Could you check a few things on this model? Use its own coordinates, in mm. A direction names the side the tool comes from. Coordinates: 2 decimals unless noted, no trailing zeros. Order: outer loops, then holes, each group sorted by start corner. A loop starts at its lowest first (then second) coordinate and runs counter-clockwise, first axis right, second up.
```python
from build123d import *

# Parameters (mm, degrees)
BASPROSKE_W         = 2.8
BASPROSKE_H         = 16
TOOTHCUT_DEPTH      = 23.8
TEETHCUTS_COUNT     = 14
BORSKE_R            = 1.5
BORE_DEPTH          = 50.0000508
SKETCH_2_R          = 4.75
SKETCH_2_R_2        = 1.5
EXTRUDE_1_DEPTH     = 7
SKETCH_3_R          = 3.25
CUT_EXTRUDE_1_DEPTH = 3.5
CHAMFER_1_SIZE      = 1.5
SKETCH_4_W          = 3
SKETCH_4_H          = 9.5
CUT_EXTRUDE_2_DEPTH = 2


with BuildPart() as part:
    # BasProSke → Base-Revolve (revolve)
    with BuildSketch(Plane(origin=(0, 0, 0), x_dir=(1, 0, 0), z_dir=(0, 1, 0)), mode=Mode.PRIVATE) as base_revolve_sk:
        with Locations((1.4, 8)):
            Rectangle(BASPROSKE_W, BASPROSKE_H)
    revolve(base_revolve_sk.sketch.rotate(Axis((-10, 0, 0), (1, 0, 0)), 180), axis=Axis((-10, 0, 0), (1, 0, 0)))

    # TooCutSke → ToothCut (cut, through all)
    with BuildSketch(Plane(origin=(0, 0, 0), x_dir=(0, 0, -1), z_dir=(1, 0, 0))):
        with BuildLine():
            ThreePointArc((1.067858192, 11.449309144), (0, 11.499), (-1.067858192, 11.449309144))
            ThreePointArc((-1.067858192, 11.449309144), (-1.641684211, 13.812780716), (-3.163375005, 15.710076503))
            ThreePointArc((-3.163375005, 15.710076503), (0, 16.0254), (3.163375005, 15.710076503))
            ThreePointArc((3.163375005, 15.710076503), (1.641684211, 13.812780716), (1.067858192, 11.449309144))
        make_face()
    toothcut = extrude(amount=TOOTHCUT_DEPTH, mode=Mode.SUBTRACT)

    # TeethCuts: ToothCut ×14 about axis
    teethcuts_axis = Axis((0, 0, 0), (1, 0, 0))
    for i in range(1, TEETHCUTS_COUNT):
        add(toothcut.rotate(teethcuts_axis, i * 360 / TEETHCUTS_COUNT), mode=Mode.SUBTRACT)

    # BorSke → Bore (cut, symmetric)
    with BuildSketch(Plane(origin=(0, 0, 0), x_dir=(0, 0, -1), z_dir=(1, 0, 0))):
        with Locations(Location((0, 0, 0), (0, 0, 180))):
            Circle(BORSKE_R)
    extrude(amount=BORE_DEPTH, both=True, mode=Mode.SUBTRACT)

    # ｽｹｯﾁ2 → ﾎﾞｽ - 押し出し1 (add)
    with BuildSketch(Plane.ZY):
        with Locations(Location((0, 0, 0), (0, 0, 180))):
            Circle(SKETCH_2_R)
        Circle(SKETCH_2_R_2, mode=Mode.SUBTRACT)
    extrude(amount=EXTRUDE_1_DEPTH)

    # ｽｹｯﾁ3 → ｶｯﾄ - 押し出し1 (cut)
    with BuildSketch(Plane(origin=(2.8, 0, 0), x_dir=(0, 0, -1), z_dir=(1, 0, 0))):
        Circle(SKETCH_3_R)
    extrude(amount=-CUT_EXTRUDE_1_DEPTH, mode=Mode.SUBTRACT)

    # 面取り1
    chamfer_1_edges = [part.edges().sort_by_distance(p)[0] for p in [
        (0, 0, 4.75),
    ]]
    chamfer(chamfer_1_edges, length=CHAMFER_1_SIZE)

    # ｽｹｯﾁ4 → ｶｯﾄ - 押し出し2 (cut)
    with BuildSketch(Plane.ZY.offset(7)):
        Rectangle(SKETCH_4_W, SKETCH_4_H)
    extrude(amount=-CUT_EXTRUDE_2_DEPTH, mode=Mode.SUBTRACT)


solid = part.part
```
Item 1: Suppose I cut it at C-C (x = -3.75). List the corners of the cut face in (y, z) for me, and give its area (3 significant figures).
Item 2: I need wall thicknesses on line 1 (Y direction, x = -3.2, z = 0); line 2 (X direction, y = -3, z = 9.5); line 3 (Y direction, x = -6, z = 2). Which ranges of each line are inside material? Lowest first, please.
Item 3: Suppose I cut it at B-B (x = -6.25). List the corners of the cut face in (y, z) for me, and give its area (3 significant figures).
Item 4: Suppose I cut it at A-A (z = 0). List the corners of the cut face in (x, y) for me.
Item 5: Thinking about a two-plate mould opening in Y: for faces 1 (the face through (1.38, 1.485, 13.782)), 2 (the face through (-6, 0, -1.5)), 3 (the face through (1.42, -15.597, 3.566)), which applies, +Y half, -Y half, draft (parallel to the pull), parting line (faces both ways), or undercut?
Item 6: Which directions (+Z, -Z, +X, -X, +Y, -Y) give clear straight access to the entire face, cutting with the end or side of a thin tool? Please do faces 4 (the face through (1.38, -4.64, 13.06)), 5 (the face through (1.38, 13.77, 1.62)), 6 (the face through (1.38, -7.318, -11.773)).
Item 7: For pin 1 Ø6 at (y, z) = (0, 0) entering from -X; pin 2 Ø2.5 at (y, z) = (-1.5, 0) entering from -X; pin 3 Ø5 at (y, z) = (0, 0) entering from +X; pin 4 Ø1.6 at (x, y) = (-6, -1.5) entering from +Z, each with a flat end and sliding along its axis, tell me the tip position at first contact or that it passes through.
Geometry results:
1. outline: circle Ø9.5 at (0, 0); hole circle Ø3 at (0, 0)
1. area: 63.8 mm2
2. line 1: y = -4.75 to -1.5, 1.5 to 4.75
2. line 2: x = 0 to 2.8
2. line 3: y = -4.31 to 4.31
3. outline: (-4.51, -1.5) arc R4.75 ccw to (4.51, -1.5) - close; (-4.51, 1.5) - (4.51, 1.5) arc R4.75 ccw to start
3. area: 42.9 mm2
4. outline: (-5, -4.75) - (-1.5, -4.75) - (0, -6.25) - (0, -11.5) - (2.8, -11.5) - (2.8, -3.25) - (-0.7, -3.25) - (-0.7, -1.5) - (-5, -1.5) - close; (-5, 1.5) - (-0.7, 1.5) - (-0.7, 3.25) - (2.8, 3.25) - (2.8, 11.5) - (0, 11.5) - (0, 6.25) - (-1.5, 4.75) - (-5, 4.75) - close
5. face 1: undercut
5. face 2: draft
5. face 3: -Y half
6. face 4: +Z, +X, -X
6. face 5: +X, -X, +Y
6. face 6: +X, -X
7. pin 1: stops at x = -7
7. pin 2: stops at x = -5
7. pin 3: stops at x = -0.7
7. pin 4: stops at z = 4.7
